Autodesk Inventor part; units mm, degrees
ref_plane "YZ Plane" through (0, 0, 0) normal (1, 0, 0) x (0, 1, 0)
ref_plane "XZ Plane" through (0, 0, 0) normal (0, 1, 0) x (-1, 0, 0)
ref_plane "XY Plane" through (0, 0, 0) normal (0, 0, 1) x (1, 0, 0)
sketch "Sketch1" plane through (0, 0, 0) normal (0, 0, 1) x (1, 0, 0)
  line L0 (0, 5.5) -> (4.7631, 2.75)
  line L1 (4.7631, 2.75) -> (4.7631, -2.75)
  line L2 (4.7631, -2.75) -> (0, -5.5)
  line L3 (0, -5.5) -> (-4.7631, -2.75)
  line L4 (-4.7631, -2.75) -> (-4.7631, 2.75)
  line L5 (-4.7631, 2.75) -> (0, 5.5)
  point P0 (0, 0)
  point P1 (0, 0)
  dimension "d0" = 11
extrude "Extrusion1" add sketch "Sketch1" against normal blind 10
sketch "Sketch3" plane through (0, 0, 0) normal (0, 0, 1) x (1, 0, 0)
  point P0 (0, 0)
  point P1 (0, 0)
hole "Hole1" at (0, 0, 0) direction (0, 0, -1) diameter 8 depth 7
thread "Thread2"
sketch "Sketch4" plane through (0, 0, -10) normal (0, 0, -1) x (-1, 0, 0)
  point P0 (0, 0)
  point P1 (0, 0)
hole "Hole2" at (0, 0, -10) direction (0, 0, 1) diameter 5 depth 5
properties part number "159"
Input: part model. Units: mm. Frame: model coordinates. A direction names the side the tool comes from. Coordinates: 2 decimals unless noted, no trailing zeros. Loops run counter-clockwise (first coordinate to the right, second up) from the corner with the lowest first, then second, coordinate; pieces in that order, holes last. Notation, with made-up numbers: M -8,11 L 4,11 A20 ccw 4,45 Z; hole C 87.5,27.25 d9. An arc over 180 degrees is marked long. Use a Markdown table: item, result. Add a question column.
1) Pin query (flat end, axial travel): P1, Ø4, axis at x = 3.5, z = -7, coming from the -Y side; P2, Ø1, axis at x = 2, z = -5.5, coming from the +Y side. Return the tip coordinate at first contact, or that it passes through.
2) Line query: L1, parallel to X at y = 0, z = -3.75; L2, parallel to X at y = 0, z = -7.25; L3, parallel to Y at x = 1, z = -9.5. Output: solid intervals per line, ascending. Write a range as from..to.
3) Draft query along X for faces 3 (the flat face through (-2, -2, -7)), 4 (the flat face through (2, -4, 0)), 5 (the flat face through (2.348, 4.144, -4.93)). Return one class per face: +X half, -X half, draft (parallel to the pull), parting line (faces both ways), or undercut.
4) Section D-D, the plane z = -2.75. Return the cut outline in (x, y).
5) Section B-B, the plane z = -7.5. Return the cut outline in (x, y).
6) Section C-C, the plane x = -1.5. Return the cut outline in (y, z), plus the area to 3 significant figures.
7) Set-up query: faces 1 (the flat face through (4.763, 0, -5)), 2 (the cylindrical face through (3.905, 0.867, -3.549)). Return all of +Z, -Z, +X, -X, +Y, -Y with unobstructed straight access to the full face (end or side cutting, diameter ignored); none if empty.
8) Section A-A, the plane y = 0. Return the cut outline in (x, z).
Answer below:
| question | item | result |
|---|---|---|
| 1 | P1 | y = -4.63 |
| 1 | P2 | y = 4.63 |
| 2 | L1 | -4.76..-4, 4..4.76 |
| 2 | L2 | -4.76..-2.5, 2.5..4.76 |
| 2 | L3 | -4.92..-2.29, 2.29..4.92 |
| 3 | face 3 | undercut |
| 3 | face 4 | draft |
| 3 | face 5 | +X half |
| 4 | outline | M -4.76,-2.75 L 0,-5.5 L 4.76,-2.75 L 4.76,2.75 L 0,5.5 L -4.76,2.75 Z; hole C 0,0 d8 |
| 5 | outline | M -4.76,-2.75 L 0,-5.5 L 4.76,-2.75 L 4.76,2.75 L 0,5.5 L -4.76,2.75 Z; hole C 0,0 d5 |
| 6 | outline | M -4.63,-10 L -2,-10 L -2,-7 L -3.71,-7 L -3.71,0 L -4.63,0 Z; M 2,-10 L 4.63,-10 L 4.63,0 L 3.71,0 L 3.71,-7 L 2,-7 Z |
| 6 | area | 28.8 mm2 |
| 7 | face 1 | +Z, -Z, +X, +Y, -Y |
| 7 | face 2 | +Z |
| 8 | outline | M -4.76,-10 L -2.5,-10 L -2.5,-7 L -4,-7 L -4,0 L -4.76,0 Z; M 2.5,-10 L 4.76,-10 L 4.76,0 L 4,0 L 4,-7 L 2.5,-7 Z |
